Can you work these out from the model? Positions are in its coordinate system, mm. Face numbers are marked on the shaded views. A direction names the side the tool comes from. Coordinates: 2 decimals unless noted, no trailing zeros. Loops run counter-clockwise (first coordinate to the right, second up) from the corner with the lowest first, then second, coordinate; pieces in that order, holes last. Notation, with made-up numbers: (26.25, 37) -> (76.25, 37) arc R16 cw to (76.25, 50) -> close; hole circle Ø4 at (54, -23). An arc over 180 degrees is marked (long way). Put each result on its own line as item: value. Start each with the question number.
Item 1: Please list where these lines run through material, in increasing order: L1, parallel to Y at x = -0.25, z = -21.5; L2, parallel to Z at x = 2.25, y = 0. Write a range as from..to.
Item 2: If we section it at B-B on z = -1: Please give me the cut outline in (x, y), plus the area to 3 significant figures.
Item 3: Will these pins go through, and if not, where does the flat tip stop? P1, Ø2, axis at x = 1, y = 2, coming from the -Z side; P2, Ø1.5, axis at y = 1, z = -9.5, coming from the +X side.
Item 4: If we section it at A-A on x = 0: Please give me the cut outline in (y, z), plus the area to 3 significant figures.
Item 5: For the marked faces 1 and 2, which set-ups out of +Z, -Z, +X, -X, +Y, -Y let a thin tool reach every point of the face, with its end or its side?
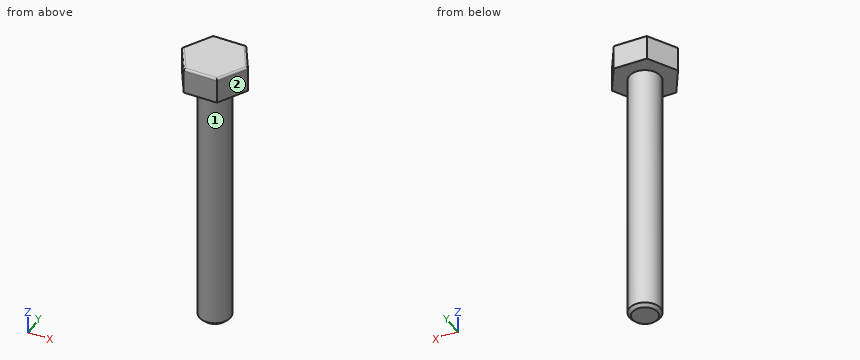
```python
from build123d import *

# Parameters (mm, degrees)
BOSS_EXTRUDE1_DEPTH = 2.5
SKETCH2_R           = 1.5
BOSS_EXTRUDE2_DEPTH = 25
CHAMFER1_SIZE       = 0.3
FILLET1_R           = 0.2


with BuildPart() as part:
    # Sketch1 → Boss-Extrude1 (new body)
    with BuildSketch(Plane.XY):
        Polygon((3.175426481, 0), (1.58771324, 2.75), (-1.58771324, 2.75), (-3.175426481, 0), (-1.58771324, -2.75), (1.58771324, -2.75), align=None)
    extrude(amount=BOSS_EXTRUDE1_DEPTH)

    # Sketch2 → Boss-Extrude2 (add)
    with BuildSketch(Plane(origin=(0, 0, 0), x_dir=(-1, 0, 0), z_dir=(0, 0, -1))):
        Circle(SKETCH2_R)
    extrude(amount=BOSS_EXTRUDE2_DEPTH)

    # Chamfer1
    chamfer1_edges = [part.edges().sort_by_distance(p)[0] for p in [
        (1.5, 0, -25),
    ]]
    chamfer(chamfer1_edges, length=CHAMFER1_SIZE)

    # Fillet1
    fillet1_edges = [part.edges().sort_by_distance(p)[0] for p in [
        (0, 2.75, 2.5),
        (-2.38156986, 1.375, 2.5),
        (-2.38156986, -1.375, 2.5),
        (0, -2.75, 2.5),
        (2.38156986, -1.375, 2.5),
        (2.38156986, 1.375, 2.5),
    ]]
    fillet(fillet1_edges, radius=FILLET1_R)


solid = part.part
```
Solutions:
1. L1: -1.48..1.48
1. L2: 0..2.5
2. outline: circle Ø3 at (0, 0)
2. area: 7.07 mm^2
3. P1: z = -24.96
3. P2: x = 1.48
4. outline: (-2.75, 0) -> (-1.5, 0) -> (-1.5, -24.7) -> (-1.2, -25) -> (1.2, -25) -> (1.5, -24.7) -> (1.5, 0) -> (2.75, 0) -> (2.75, 2.3) arc R0.2 ccw to (2.55, 2.5) -> (-2.55, 2.5) arc R0.2 ccw to (-2.75, 2.3) -> close
4. area: 88.6 mm^2
5. face 1: -Z
5. face 2: +Z, -Z, +X, -Y
